```python
from build123d import *

# Parameters (mm, degrees)
SKETCH_R        = 5
PAD_DEPTH       = 4
SKETCH001_R     = 1.7
POCKET_DEPTH    = 4.001
SKETCH002_R     = 2.95
POCKET001_DEPTH = 3


with BuildPart() as part:
    # Sketch → Pad (new body)
    with BuildSketch(Plane.XY):
        with BuildLine():
            Line((-7.200521, 3.25), (-15, 3.25))
            Line((-15, 3.25), (-15, -3.25))
            Line((-15, -3.25), (-7.200521, -3.25))
            ThreePointArc((-7.200521, -3.25), (0, -7.9), (7.200521, -3.25))
            Line((15, -3.25), (7.200521, -3.25))
            Line((15, 3.25), (15, -3.25))
            Line((7.200521, 3.25), (15, 3.25))
            ThreePointArc((7.200521, 3.25), (0, 7.9), (-7.200521, 3.25))
        make_face()
        Circle(SKETCH_R, mode=Mode.SUBTRACT)
    extrude(amount=PAD_DEPTH)

    # Sketch001 (on Face10 of Pad) → Pocket (cut, through all)
    with BuildSketch(Plane(origin=(0, 0, 0), x_dir=(1, 0, 0), z_dir=(0, 0, -1))):
        with Locations((11, 0)):
            Circle(SKETCH001_R)
        with Locations((-11, 0)):
            Circle(SKETCH001_R)
    extrude(amount=-POCKET_DEPTH, mode=Mode.SUBTRACT)

    # Sketch002 (on Face5 of Pocket) → Pocket001 (cut)
    with BuildSketch(Plane.XY.offset(4)):
        with Locations((11, 0)):
            Circle(SKETCH002_R)
        with Locations((-11, 0)):
            Circle(SKETCH002_R)
    extrude(amount=-POCKET001_DEPTH, mode=Mode.SUBTRACT)


solid = part.part
```
The listing builds one solid part. Answer for the finished solid, in the listing's coordinates (mm). A direction names the side the tool comes from. Coordinates: 2 decimals unless noted, no trailing zeros. Write each loop counter-clockwise with the first axis right and the second up, starting at its lowest first coordinate (ties: lowest second). Pieces come first, ordered by that corner, then holes. Notation, with made-up numbers: (51.5, 76.25) -> (104.5, 76.25) arc R18 cw to (104.5, 92.25) -> close; hole circle Ø9 at (87.25, -4.75). An arc over 180 degrees is marked (long way). Write each question's results on one line, items separated by ' | '. Start each with the question number.
1) A tool of negligible diameter and unlimited length cuts with its end or side. For faces 5 (the flat face through (-11, -2, 1)), 6 (the flat face through (-11, 3.25, 2)), 7 (the flat face through (11, 3.25, 2)), 8 (the flat face through (11, -3.25, 2)), 9 (the cylindrical face through (12.57, 0.65, 0.49)), from which of +Z, -Z, +X, -X, +Y, -Y can it reach the whole face along a straight path? Write none if from no direction.
2) A cutting plane is placed at D-D (z = 0.4). Determine the outline of the cut face in (x, y).
3) Flat-ended cylindrical pins translate along their axes: pin 1 Ø3 at (x, y) = (-10.5, 0) entering from +Z; pin 2 Ø2 at (x, z) = (-11, 2) entering from -Y. Find the tip coordinate at first contact, or state that the pin passes through.
4) Straight lines are drawn through the part: probe 1 along X at (y, z) = (1.5, 1.1); probe 2 along Y at (x, z) = (11, 3.3); probe 3 along X at (y, z) = (-1.75, 1.8). For each, find the intervals that lie inside material, in ascending order.
5) For a pull along X with two mould halves and no side action, classify faces 1 (the cylindrical face through (8.053, 0.13, 2.521)), 2 (the flat face through (-11, -3.25, 2)), 3 (the cylindrical face through (-1.08, -4.88, 1.97)), 4 (the cylindrical face through (-0.1, -7.9, 2)) as +X half, -X half, draft (parallel to the pull), parting line (faces both ways), or undercut.
6) A cutting plane is placed at B-B (y = 0). Determine the outline of the cut face in (x, z).
7) A cutting plane is placed at C-C (x = 0). Determine the outline of the cut face in (y, z).
8) A cutting plane is placed at A-A (z = 2.45). Determine the outline of the cut face in (x, y), then the cut area to 3 significant figures.
Values follow:
1) face 5: +Z | face 6: +Z, -Z, -X, +Y | face 7: +Z, -Z, +X, +Y | face 8: +Z, -Z, +X, -Y | face 9: +Z, -Z
2) outline: (-15, -3.25) -> (-7.2, -3.25) arc R7.9 ccw to (7.2, -3.25) -> (15, -3.25) -> (15, 3.25) -> (7.2, 3.25) arc R7.9 ccw to (-7.2, 3.25) -> (-15, 3.25) -> close; hole circle Ø3.4 at (-11, 0); hole circle Ø10 at (0, 0); hole circle Ø3.4 at (11, 0)
3) pin 1: z = 1 | pin 2: y = -3.25
4) probe 1: -15 to -13.54, -8.46 to -4.77, 4.77 to 8.46, 13.54 to 15 | probe 2: -3.25 to -2.95, 2.95 to 3.25 | probe 3: -15 to -13.37, -8.63 to -4.68, 4.68 to 8.63, 13.37 to 15
5) face 1: undercut | face 2: draft | face 3: undercut | face 4: parting line
6) outline: (-15, 0) -> (-12.7, 0) -> (-12.7, 1) -> (-13.95, 1) -> (-13.95, 4) -> (-15, 4) -> close; (-9.3, 0) -> (-5, 0) -> (-5, 4) -> (-8.05, 4) -> (-8.05, 1) -> (-9.3, 1) -> close; (5, 0) -> (9.3, 0) -> (9.3, 1) -> (8.05, 1) -> (8.05, 4) -> (5, 4) -> close; (12.7, 0) -> (15, 0) -> (15, 4) -> (13.95, 4) -> (13.95, 1) -> (12.7, 1) -> close
7) outline: (-7.9, 0) -> (-5, 0) -> (-5, 4) -> (-7.9, 4) -> close; (5, 0) -> (7.9, 0) -> (7.9, 4) -> (5, 4) -> close
8) outline: (-15, -3.25) -> (-7.2, -3.25) arc R7.9 ccw to (7.2, -3.25) -> (15, -3.25) -> (15, 3.25) -> (7.2, 3.25) arc R7.9 ccw to (-7.2, 3.25) -> (-15, 3.25) -> close; hole circle Ø5.9 at (-11, 0); hole circle Ø10 at (0, 0); hole circle Ø5.9 at (11, 0) | area: 158 mm²
